```python
from build123d import *

# Parameters (mm, degrees)
SKETCH1_R           = 6
BOSS_EXTRUDE1_DEPTH = 10
CUT_EXTRUDE1_DEPTH  = 6
CUT_EXTRUDE2_DEPTH  = 5


with BuildPart() as part:
    # Sketch1 → Boss-Extrude1 (new body)
    with BuildSketch(Plane(origin=(0, 0, 0), x_dir=(1, 0, 0), z_dir=(0, 1, 0))):
        with Locations(Location((0, 0, 0), (0, 0, 270))):
            Circle(SKETCH1_R)
    extrude(amount=BOSS_EXTRUDE1_DEPTH)

    # Sketch3 → Cut-Extrude1 (cut)
    with BuildSketch(Plane.XZ):
        with BuildLine():
            Line((2.5, -2.485080482), (2.5, 2.485080482))
            ThreePointArc((2.5, 2.485080482), (0, 3.525), (-2.5, 2.485080482))
            Line((-2.5, 2.485080482), (-2.5, -2.485080482))
            ThreePointArc((-2.5, -2.485080482), (0, -3.525), (2.5, -2.485080482))
        make_face()
    extrude(amount=-CUT_EXTRUDE1_DEPTH, mode=Mode.SUBTRACT)

    # Sketch2 → Cut-Extrude2 (cut)
    with BuildSketch(Plane(origin=(0, 10, 0), x_dir=(1, 0, 0), z_dir=(0, 1, 0))):
        with BuildLine():
            Line((1.95, -1.643167673), (1.95, 1.643167673))
            ThreePointArc((1.95, 1.643167673), (0, 2.55), (-1.95, 1.643167673))
            Line((-1.95, 1.643167673), (-1.95, -1.643167673))
            ThreePointArc((-1.95, -1.643167673), (0, -2.55), (1.95, -1.643167673))
        make_face()
    extrude(amount=-CUT_EXTRUDE2_DEPTH, mode=Mode.SUBTRACT)


solid = part.part
```
Geometry: final body of the model. Coordinates: model frame, mm. A direction names the side the tool comes from. Give positions to 0.01 mm unless a question says otherwise; leave off trailing zeros. Write each loop counter-clockwise with the first axis right and the second up, starting at its lowest first coordinate (ties: lowest second). Pieces come first, ordered by that corner, then holes.
1. Section query D-D, the plane z = 3. Return loops of the section in (x, y), then the cut area to 3 significant figures.
2. Reachability of faces 4 (the cylindrical face through (-0.03, 8.03, 2.55)), 5 (the flat face through (-2.5, 3, 0)), 6 (the flat face through (0, 10, 3)) from +Z, -Z, +X, -X, +Y, -Y: full face, straight path, thin tool, end or side. Return the list, or none.
3. Section query A-A, the plane x = 0. Return loops of the section in (y, z) (3 decimals), then the cut area to 3 significant figures.
4. Section query B-B, the plane z = 0. Return loops of the section in (x, y), then the cut area to 3 significant figures.
5. Draft query along X for faces 1 (the flat face through (2.5, 3, 0)), 2 (the flat face through (-3, 0, 0)), 3 (the cylindrical face through (1.802, 4.93, 5.723)). Return one class per face: released by +X, released by -X, zero draft, split by the parting line, or undercut.
6. Pin query (flat end, axial travel): P1, Ø2, axis at y = 1, z = -4, coming from the -X side; P2, Ø4, axis at x = -3, y = 3, coming from the -Z side. Return the tip coordinate at first contact, or that it passes through.
7. Line query: probe 1 along Z at (x, y) = (-1.75, 2.75); probe 2 along Z at (x, y) = (-0.25, 4.5); probe 3 along Y at (x, z) = (-0.5, -2.75). Output: solid intervals per line, ascending.
8. Section query C-C, the plane y = 9. Return loops of the section in (x, z).
Computed:
1. outline: (-5.2, 0) - (-1.85, 0) - (-1.85, 6) - (1.85, 6) - (1.85, 0) - (5.2, 0) - (5.2, 10) - (-5.2, 10) - close
1. area: 81.7 mm2
2. face 4: +Y, -Y
2. face 5: -Y
2. face 6: +Z, -Z, +X, -X, +Y
3. outline: (0, -6) - (10, -6) - (10, -2.55) - (6, -2.55) - (6, -3.525) - (0, -3.525) - close; (0, 3.525) - (6, 3.525) - (6, 2.55) - (10, 2.55) - (10, 6) - (0, 6) - close
3. area: 57.3 mm2
4. outline: (-6, 0) - (-2.5, 0) - (-2.5, 6) - (-1.95, 6) - (-1.95, 10) - (-6, 10) - close; (1.95, 6) - (2.5, 6) - (2.5, 0) - (6, 0) - (6, 10) - (1.95, 10) - close
4. area: 74.4 mm2
5. face 1: undercut
5. face 2: zero draft
5. face 3: split by the parting line
6. P1: stops at x = -5.2
6. P2: stops at z = -5.92
7. probe 1: z = -5.74 to -3.06, 3.06 to 5.74
7. probe 2: z = -5.99 to -3.52, 3.52 to 5.99
7. probe 3: y = 6 to 10
8. outline: circle Ø12 at (0, 0); hole (-1.95, -1.64) arc R2.55 ccw to (1.95, -1.64) - (1.95, 1.64) arc R2.55 ccw to (-1.95, 1.64) - close
